Source: CAD feature listing. Evaluate the final solid. Frame: model axes, mm. Face numbers are marked on the shaded views. A direction names the side the tool comes from. Give positions to 0.01 mm unless a question says otherwise; leave off trailing zeros. Loops run counter-clockwise (first coordinate to the right, second up) from the corner with the lowest first, then second, coordinate; pieces in that order, holes last. Notation, with made-up numbers: (84, 11) -> (141, 11) arc R21 ccw to (141, 50) -> close; hole circle Ø7 at (5, 36.25). An arc over 180 degrees is marked (long way). Return JSON: item names as keys, results as strings. Group by question number.
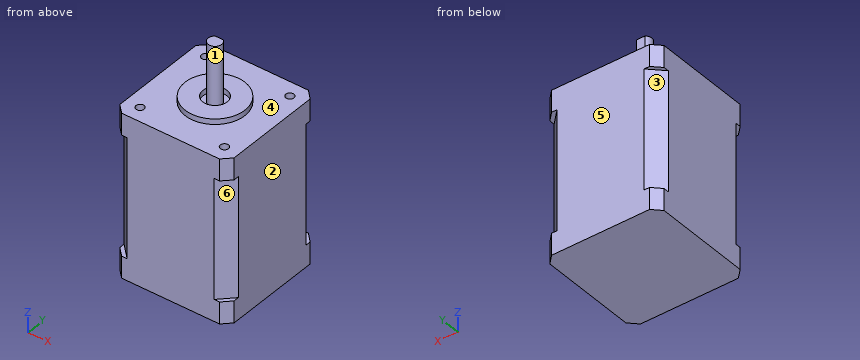
```python
from build123d import *

# Parameters (mm, degrees)
SALIENTE_EXTRUIR1_DEPTH = 44
SALIENTE_EXTRUIR2_DEPTH = 8
SALIENTE_EXTRUIR3_DEPTH = 8
CROQUIS4_R              = 11
CROQUIS4_R_2            = 4.5
SALIENTE_EXTRUIR4_DEPTH = 2
CROQUIS5_R              = 2.5
SALIENTE_EXTRUIR5_DEPTH = 22
CORTAR_EXTRUIR1_START   = -15
CORTAR_EXTRUIR1_DEPTH   = 15
CROQUIS7_R              = 1.5
CORTAR_EXTRUIR2_DEPTH   = 4


with BuildPart() as part:
    # Croquis1 → Saliente-Extruir1 (new body)
    with BuildSketch(Plane.XY):
        Polygon((-21, 16), (-16, 21), (16, 21), (21, 16), (21, -16), (16, -21), (-16, -21), (-21, -16), align=None)
    extrude(amount=SALIENTE_EXTRUIR1_DEPTH)

    # Croquis2 → Saliente-Extruir2 (add)
    with BuildSketch(Plane.XY.offset(44)):
        Polygon((-21, 18), (-18, 21), (18, 21), (21, 18), (21, -18), (18, -21), (-18, -21), (-21, -18), align=None)
    extrude(amount=SALIENTE_EXTRUIR2_DEPTH)

    # Croquis3 → Saliente-Extruir3 (add)
    with BuildSketch(Plane(origin=(0, 0, 0), x_dir=(-1, 0, 0), z_dir=(0, 0, -1))):
        Polygon((-21, 18), (-18, 21), (18, 21), (21, 18), (21, -18), (18, -21), (-18, -21), (-21, -18), align=None)
    extrude(amount=SALIENTE_EXTRUIR3_DEPTH)

    # Croquis4 → Saliente-Extruir4 (add)
    with BuildSketch(Plane.XY.offset(52)):
        with Locations(Location((0, 0, 0), (0, 0, 180))):
            Circle(CROQUIS4_R)
        Circle(CROQUIS4_R_2, mode=Mode.SUBTRACT)
    extrude(amount=SALIENTE_EXTRUIR4_DEPTH)

    # Croquis5 → Saliente-Extruir5 (add)
    with BuildSketch(Plane.XY.offset(52)):
        with Locations(Location((0, 0, 0), (0, 0, 180))):
            Circle(CROQUIS5_R)
    extrude(amount=SALIENTE_EXTRUIR5_DEPTH)

    # Croquis6 → Cortar-Extruir1 (cut)
    with BuildSketch(Plane.XY.offset(74).offset(CORTAR_EXTRUIR1_START)):
        with BuildLine():
            Line((-1.5, 2), (1.5, 2))
            ThreePointArc((1.5, 2), (0, 2.5), (-1.5, 2))
        make_face()
    extrude(amount=CORTAR_EXTRUIR1_DEPTH, mode=Mode.SUBTRACT)

    # Croquis7 → Cortar-Extruir2 (cut)
    with BuildSketch(Plane.XY.offset(52)):
        with Locations((-15.5, 15.5)):
            Circle(CROQUIS7_R)
        with Locations((15.5, 15.5)):
            Circle(CROQUIS7_R)
        with Locations((15.5, -15.5)):
            Circle(CROQUIS7_R)
        with Locations((-15.5, -15.5)):
            Circle(CROQUIS7_R)
    extrude(amount=-CORTAR_EXTRUIR2_DEPTH, mode=Mode.SUBTRACT)


solid = part.part
```
1) Reachability of the marked faces 1, 2 and 3 from +Z, -Z, +X, -X, +Y, -Y: full face, straight path, thin tool, end or side. Return the list, or none.
2) Cut plane A-A on z = 25.5. Return loops of the section in (x, y), then the cut area to 3 significant figures.
3) Contact query for flat-ended pins moving along their axis: P1, Ø8, axis at x = -11, y = -8, coming from the +Z side; P2, Ø1.5, axis at x = -15, y = 16, coming from the +Z side; P3, Ø1.5, axis at x = -0.5, z = 67, coming from the +Y side. Output: stop coordinate, or through.
4) Cut plane B-B on y = 0. Return loops of the section in (x, z).
5) Material intervals for line 1 (Y direction, x = 0, z = 53.5); line 2 (Y direction, x = -15, z = 50); line 3 (Z direction, x = 11, y = 1), sorted ascending.
6) Cut plane D-D on z = 62. Return loops of the section in (x, y).
7) Cut plane C-C on x = 0. Return loops of the section in (y, z).
8) Mould query, pull axis Z, two halves, no side actions, for the marked faces 4, 5 and 6. Classes: released by +Z, released by -Z, zero draft, split by the parting line, or undercut.
Calculated:
{
 "1": {"face 1": "+Z", "face 2": "+Z, -Z, +X, +Y, -Y", "face 3": "-X, +Y"},
 "2": {"outline": "(-21, -16) -> (-16, -21) -> (16, -21) -> (21, -16) -> (21, 16) -> (16, 21) -> (-16, 21) -> (-21, 16) -> close", "area": "1,710 mm2"},
 "3": {"P1": "z = 54", "P2": "z = 48", "P3": "y = 2"},
 "4": {"outline": "(-21, -8) -> (21, -8) -> (21, 52) -> (11, 52) -> (11, 54) -> (4.5, 54) -> (4.5, 52) -> (2.5, 52) -> (2.5, 74) -> (-2.5, 74) -> (-2.5, 52) -> (-4.5, 52) -> (-4.5, 54) -> (-11, 54) -> (-11, 52) -> (-21, 52) -> close"},
 "5": {"line 1": "-11 to -4.5, -2.5 to 2.5, 4.5 to 11", "line 2": "-21 to -16.91, -14.09 to 14.09, 16.91 to 21", "line 3": "-8 to 52"},
 "6": {"outline": "(-1.5, 2) arc R2.5 ccw (long way) to (1.5, 2) -> close"},
 "7": {"outline": "(-21, -8) -> (21, -8) -> (21, 52) -> (11, 52) -> (11, 54) -> (4.5, 54) -> (4.5, 52) -> (2.5, 52) -> (2.5, 59) -> (2, 59) -> (2, 74) -> (-2.5, 74) -> (-2.5, 52) -> (-4.5, 52) -> (-4.5, 54) -> (-11, 54) -> (-11, 52) -> (-21, 52) -> close"},
 "8": {"face 4": "released by +Z", "face 5": "zero draft", "face 6": "undercut"}
}
